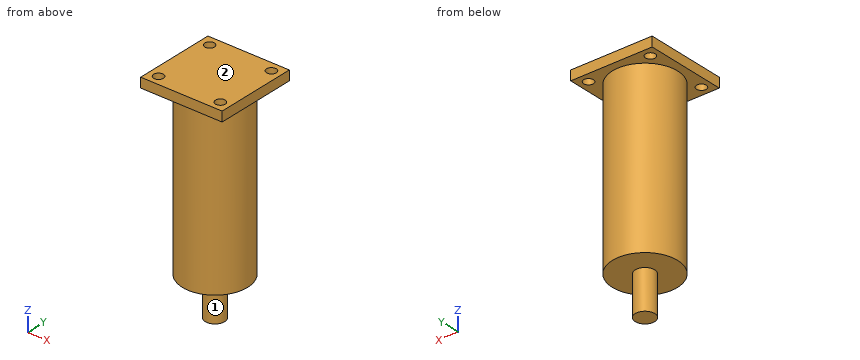
```python
from build123d import *

# Parameters (mm, degrees)
SKETCH_2_W          = 25
SKETCH_2_H          = 25
EXTRUDE_1_DEPTH     = 3
SKETCH_3_R          = 1.5
CUT_EXTRUDE_2_DEPTH = 4
EXTRUDE_START       = -3
SKETCH_4_R          = 10
EXTRUDE_2_DEPTH     = 52
SKETCH_5_R          = 3
EXTRUDE_3_DEPTH     = 12


with BuildPart() as part:
    # 草图2 → 凸台-拉伸1 (new body)
    with BuildSketch(Plane.XY):
        with Locations((12.5, -12.5)):
            Rectangle(SKETCH_2_W, SKETCH_2_H)
    extrude(amount=EXTRUDE_1_DEPTH)

    # 草图3 → 切除-拉伸2 (cut, through all)
    with BuildSketch(Plane(origin=(0, 0, 0), x_dir=(-1, 0, 0), z_dir=(0, 0, -1))):
        with Locations((-22, -3)):
            Circle(SKETCH_3_R)
        with Locations((-3, -3)):
            Circle(SKETCH_3_R)
        with Locations((-3, -22)):
            Circle(SKETCH_3_R)
        with Locations((-22, -22)):
            Circle(SKETCH_3_R)
    extrude(amount=-CUT_EXTRUDE_2_DEPTH, mode=Mode.SUBTRACT)

    # 草图4 → 凸台-拉伸2 (add)
    with BuildSketch(Plane.XY.offset(3).offset(EXTRUDE_START)):
        with Locations((12.5, -12.5)):
            Circle(SKETCH_4_R)
    extrude(amount=-EXTRUDE_2_DEPTH)

    # 草图5 → 凸台-拉伸3 (add)
    with BuildSketch(Plane(origin=(0, 0, -52), x_dir=(-1, 0, 0), z_dir=(0, 0, -1))):
        with Locations((-12.5, -12.5)):
            Circle(SKETCH_5_R)
    extrude(amount=EXTRUDE_3_DEPTH)


solid = part.part
```
Part model, mm, in its own coordinate system. Face numbers are marked on the shaded views. A direction names the side the tool comes from. Give positions to 0.01 mm unless a question says otherwise; leave off trailing zeros. Order: outer loops, then holes, each group sorted by start corner. A loop starts at its lowest first (then second) coordinate and runs counter-clockwise, first axis right, second up. Notation, with made-up numbers: (63.5, 65) - (122.5, 65) arc R29 cw to (122.5, 102) - close; hole circle Ø5 at (25, -21.5). An arc over 180 degrees is marked (long way). Use one line per item in the form item = value.
Item 1: Slice it at C-C on z = -43.5. Give the cut face in (x, y), and give its area (3 significant figures).
Solution:
outline = circle Ø20 at (12.5, -12.5)
area = 314 mm2
Item 2: Slice it at A-A on x = 18.5. Give the cut face in (y, z), and give its area (3 significant figures).
Solution:
outline = (-25, 0) - (-20.5, 0) - (-20.5, -52) - (-4.5, -52) - (-4.5, 0) - (0, 0) - (0, 3) - (-25, 3) - close
area = 907 mm2
Item 3: Which spindle directions (+Z, -Z, +X, -X, +Y, -Y) get a long thin tool onto all of the face, cutting with end or side? Do the marked faces 1 and 2. Say none if no direction does.
Solution:
face_1 = -Z
face_2 = +Z, +X, -X, +Y, -Y
Item 4: Slice it at B-B on y = -12.5. Give the cut face in (x, z).
Solution:
outline = (0, 0) - (2.5, 0) - (2.5, -52) - (9.5, -52) - (9.5, -64) - (15.5, -64) - (15.5, -52) - (22.5, -52) - (22.5, 0) - (25, 0) - (25, 3) - (0, 3) - close
Item 5: Probe probe 1 along Y at (x, z) = (22, 1.6); probe 2 along Z at (x, y) = (20.5, -18); probe 3 along X at (y, z) = (-12.25, -10). List the from-to ranges inside material, lowest first. Write a range as from..to.
Solution:
probe_1 = -25..-23.5, -20.5..-4.5, -1.5..0
probe_2 = -52..3
probe_3 = 2.5..22.5
Item 6: Pin check, flat tips, straight feed: pin 1 Ø4 at (x, z) = (12, -41) entering from -Y; pin 2 Ø1 at (x, z) = (21, -16) entering from -Y; pin 3 Ø1.5 at (y, z) = (-9, -31.5) entering from -X; pin 4 Ø2.5 at (x, y) = (3, -3) entering from -Z. Stop position of each tip, or through.
Solution:
pin_1 = -22.5
pin_2 = -18.5
pin_3 = 2.89
pin_4 = through
Item 7: Slice it at D-D on y = -19.25. Give the cut face in (x, z), and give its area (3 significant figures).
Solution:
outline = (0, 0) - (5.12, 0) - (5.12, -52) - (19.88, -52) - (19.88, 0) - (25, 0) - (25, 3) - (0, 3) - close
area = 842 mm2
